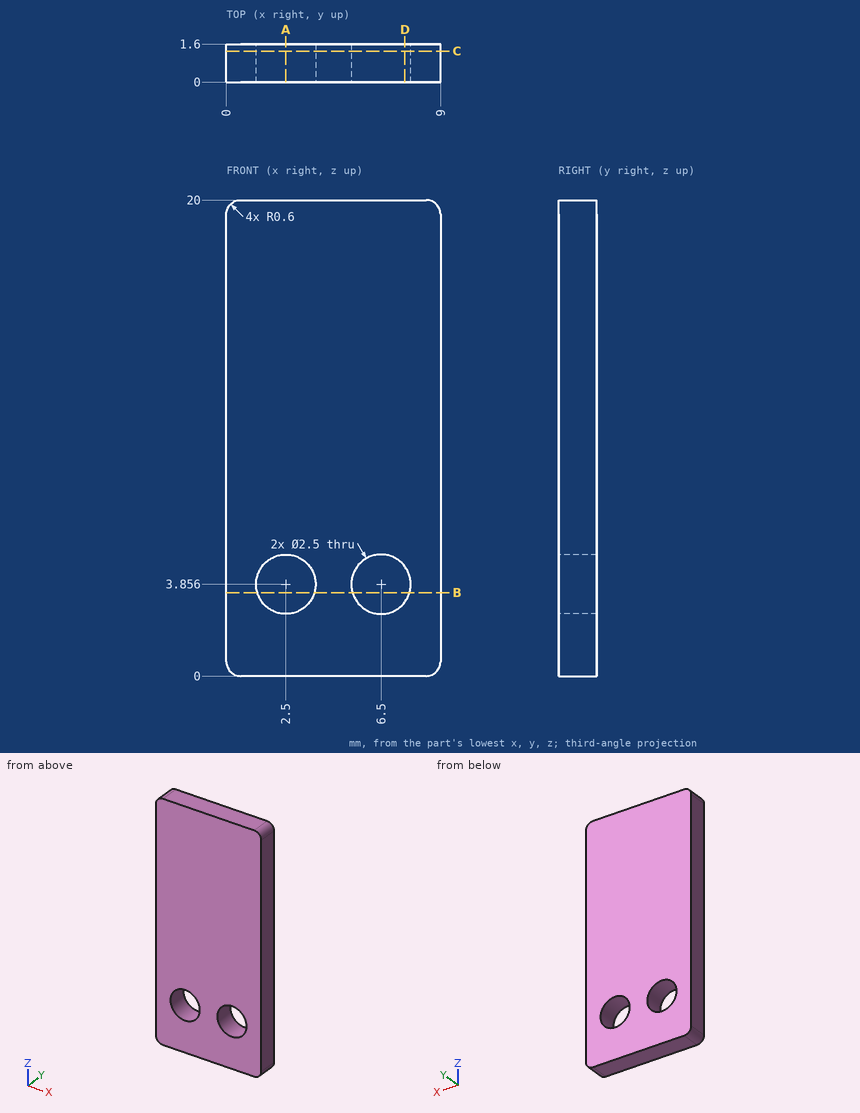
Study the drawing (mm; zero at the part's minimum x, y, z) and answer. Coordinates: 2 decimals unless noted, no trailing zeros. Write each loop counter-clockwise with the first axis right and the second up, starting at its lowest first coordinate (ties: lowest second). Pieces come first, ordered by that corner, then holes. Notation, with made-up numbers: M -35,74 L -11,74 A36 ccw -11,108 Z; hole C 23.5,56 d5. An arc over 180 degrees is marked long. Use one line per item in the form item = value.
Item 1: Find section C-C, the plane y = 1.3. Give the number of separate pieces and of enclosed holes in the cut face, plus the area to 3 significant figures.
Model answer:
separate_pieces = 1
enclosed_holes = 2
area = 170 mm2
Item 2: Find section D-D, the plane x = 7.5. Give the vertices of the cut face in (y, z) (1 decimal).
Model answer:
outline = M 0,0 L 1.6,0 L 1.6,3.1 L 0,3.1 Z; M 0,4.6 L 1.6,4.6 L 1.6,20 L 0,20 Z
Item 3: Find section A-A, the plane x = 2.5. Give the vertices of the cut face in (y, z) (1 decimal).
Model answer:
outline = M 0,0 L 1.6,0 L 1.6,2.6 L 0,2.6 Z; M 0,5.1 L 1.6,5.1 L 1.6,20 L 0,20 Z
Item 4: Given P1, Ø1.5, axis at x = 2.5, z = 3.86, coming from the +Y side, flat-ended and moving along its own axis, determine where the tip first touches the part or whether it passes through.
Model answer:
P1 = through
Item 5: Find section B-B, the plane z = 3.5. Give the vertices of the cut face in (x, y).
Model answer:
outline = M 0,0 L 1.3,0 L 1.3,1.6 L 0,1.6 Z; M 3.7,0 L 5.3,0 L 5.3,1.6 L 3.7,1.6 Z; M 7.7,0 L 9,0 L 9,1.6 L 7.7,1.6 Z
Item 6: Find the intervals of material crossed by probe 1 along Z at (x, y) = (6.5, 0.7) (1 decimal); probe 2 along X at (y, z) = (0.2, 3); probe 3 along X at (y, z) = (0.95, 5) (1 decimal), in increasing order.
Model answer:
probe_1 = 0 to 2.6, 5.1 to 20
probe_2 = 0 to 1.59, 3.41 to 5.59, 7.41 to 9
probe_3 = 0 to 2, 3 to 6, 7 to 9
